Job drawing, mm, ordinate dimensions from the low corner. One solid piece. A direction names the side the tool comes from. Round coordinates to 2 decimals unless told otherwise and drop trailing zeros. Write each loop counter-clockwise with the first axis right and the second up, starting at its lowest first coordinate (ties: lowest second). Pieces come first, ordered by that corner, then holes. Notation, with made-up numbers: (-8.5, 57) - (24.5, 57) arc R23 ccw to (24.5, 80) - close; hole circle Ø11 at (70, -8). An arc over 180 degrees is marked (long way). Write each question's results on one line, items separated by ' | '.
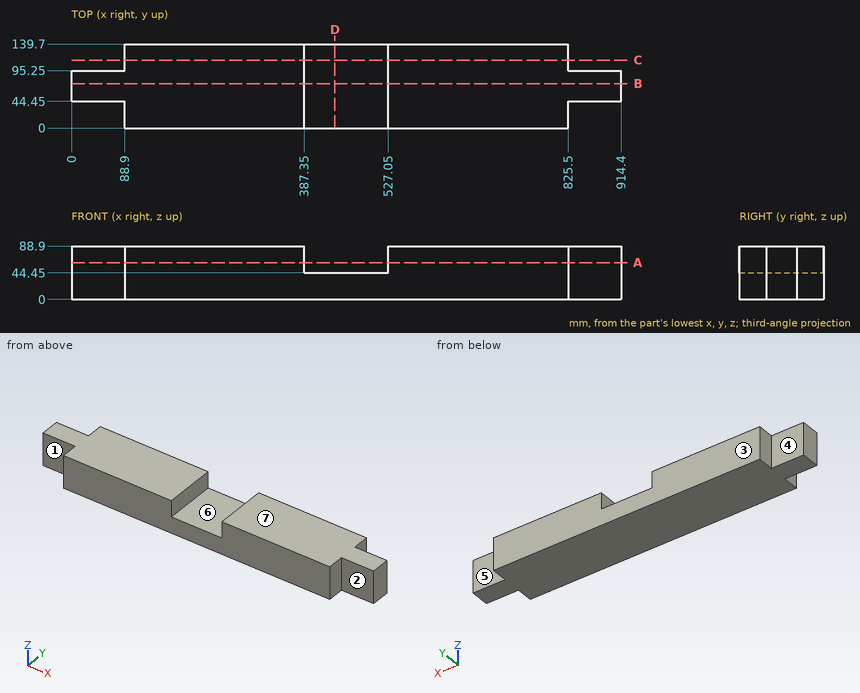
(1) Drill centre lines: probe 1 along X at (y, z) = (12, 77); probe 2 along X at (y, z) = (87.5, 66); probe 3 along X at (y, z) = (112, 36.5). Where is each one in solid material? Low to high. Write a range as [from, to].
Worked answers:
probe 1: x = [88.9, 387.35], [527.05, 825.5] | probe 2: x = [0, 387.35], [527.05, 914.4] | probe 3: x = [88.9, 825.5]
(2) Slice it at D-D, the plane x = 438. Write the cut outline in (y, z).
Worked answers:
outline: (0, 0) - (139.7, 0) - (139.7, 44.45) - (0, 44.45) - close
(3) Tool access for the marked faces 1, 2, 3, 4 and 5: list every direction of +Z, -Z, +X, -X, +Y, -Y with a clear straight run to the whole face (end or side of a thin tool).
Worked answers:
face 1: +Z, -Z, -X, -Y | face 2: +Z, -Z, +X, -Y | face 3: +Z, -Z, +X, -X, +Y | face 4: +Z, -Z, -X, +Y | face 5: +Z, -Z, +X, +Y
(4) Flat gauge pins, fed straight in: pin 1 Ø13.5 at (y, z) = (13.5, 32.5) entering from +X; pin 2 Ø13.5 at (y, z) = (112, 33) entering from -X; pin 3 Ø1.5 at (x, y) = (463, 105) entering from +Z. Where does each tip first touch, or does it go through?
Worked answers:
pin 1: stops at x = 825.5 | pin 2: stops at x = 88.9 | pin 3: stops at z = 44.45
(5) Two-plate mould, pull along X, no slides. Class the marked faces 6 and 7: released by +X, released by -X, zero draft, split by the parting line, or undercut.
Worked answers:
face 6: undercut | face 7: zero draft
(6) Slice it at A-A, the plane z = 61.5. Write the cut outline in (x, y), and give its area (3 significant figures).
Worked answers:
outline: (0, 44.45) - (88.9, 44.45) - (88.9, 0) - (387.35, 0) - (387.35, 139.7) - (88.9, 139.7) - (88.9, 95.25) - (0, 95.25) - close; (527.05, 0) - (825.5, 0) - (825.5, 44.45) - (914.4, 44.45) - (914.4, 95.25) - (825.5, 95.25) - (825.5, 139.7) - (527.05, 139.7) - close | area: 92,400 mm2
(7) Slice it at B-B, the plane y = 74. Write the cut outline in (x, z).
Worked answers:
outline: (0, 0) - (914.4, 0) - (914.4, 88.9) - (527.05, 88.9) - (527.05, 44.45) - (387.35, 44.45) - (387.35, 88.9) - (0, 88.9) - close
(8) Slice it at C-C, the plane y = 113. Write the cut outline in (x, z).
Worked answers:
outline: (88.9, 0) - (825.5, 0) - (825.5, 88.9) - (527.05, 88.9) - (527.05, 44.45) - (387.35, 44.45) - (387.35, 88.9) - (88.9, 88.9) - close
